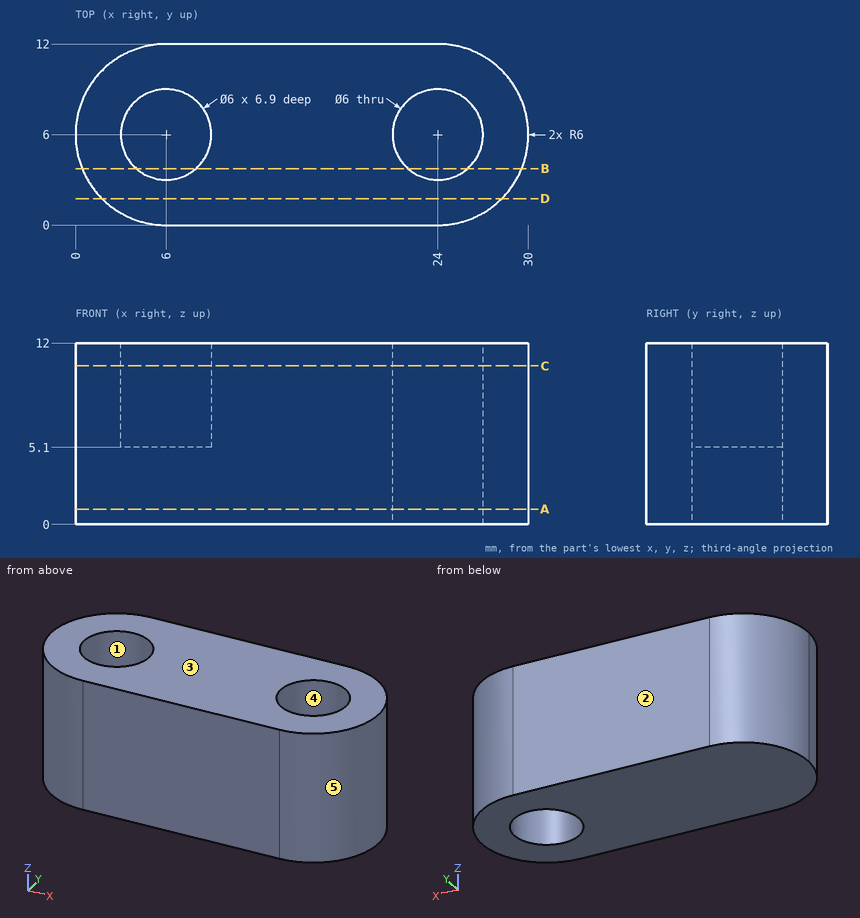
Could you check a few things on this drawing? It's one solid part, dimensions in mm from its lowest x, y, z. A direction names the side the tool comes from. Give positions to 0.01 mm unless a question says otherwise; leave off trailing zeros. Loops run counter-clockwise (first coordinate to the right, second up) from the corner with the lowest first, then second, coordinate; pieces in that order, holes last. Notation, with made-up numbers: M -34,-20.5 L 1,-20.5 A29 cw 1,10.5 Z; hole C 80.25,35.25 d11. An arc over 180 degrees is marked long. Answer as a JSON object with one key per item and string values.
Q1. For the marked faces 1 and 2, which set-ups out of +Z, -Z, +X, -X, +Y, -Y let a thin tool reach every point of the face, with its end or its side?
Values found:
{"face 1": "+Z", "face 2": "+Z, -Z, +X, -X, +Y"}
Q2. If we mould it in two halves opening along X, with no side actions, what happens to the marked faces 3, 4 and 5? For each: pulls with the +X half, pulls with the -X half, needs draft (parallel to the pull), parting line crosses it, or undercut.
Values found:
{"face 3": "needs draft", "face 4": "undercut", "face 5": "pulls with the +X half"}
Q3. If I drill on probe 1 along X at (y, z) = (3.75, 10); probe 2 along X at (y, z) = (6.5, 9); probe 3 along X at (y, z) = (5.75, 4.5), over which ranges is the centre line in solid material (lowest first)? Write a range as [from, to].
Values found:
{"probe 1": "x = [0.44, 4.02], [7.98, 22.02], [25.98, 29.56]", "probe 2": "x = [0.02, 3.04], [8.96, 21.04], [26.96, 29.98]", "probe 3": "x = [0.01, 21.01], [26.99, 29.99]"}
Q4. Suppose I cut it at B-B, the plane y = 3.75. List the corners of the cut face in (x, z) for me.
Values found:
{"outline": "M 0.44,0 L 22.02,0 L 22.02,12 L 7.98,12 L 7.98,5.1 L 4.02,5.1 L 4.02,12 L 0.44,12 Z; M 25.98,0 L 29.56,0 L 29.56,12 L 25.98,12 Z"}
Q5. For P1, Ø1, axis at y = 4.5, z = 9, coming from the +X side; P2, Ø5.5, axis at x = 24, y = 6, coming from the -Z side, each with a flat end and sliding along its axis, tell me the tip position at first contact or that it passes through.
Values found:
{"P1": "stops at x = 29.92", "P2": "passes through"}
Q6. Suppose I cut it at C-C, the plane z = 10.5. List the corners of the cut face in (x, y) for me, plus the area to 3 significant figures.
Values found:
{"outline": "M 0,6 A6 ccw 6,0 L 24,0 A6 ccw 24,12 L 6,12 A6 ccw Z; hole C 6,6 d6; hole C 24,6 d6", "area": "273 mm²"}
Q7. Suppose I cut it at A-A, the plane z = 1. List the corners of the cut face in (x, y) for me.
Values found:
{"outline": "M 0,6 A6 ccw 6,0 L 24,0 A6 ccw 24,12 L 6,12 A6 ccw Z; hole C 24,6 d6"}
Q8. Suppose I cut it at D-D, the plane y = 1.75. List the corners of the cut face in (x, z) for me.
Values found:
{"outline": "M 1.76,0 L 28.24,0 L 28.24,12 L 1.76,12 Z"}
